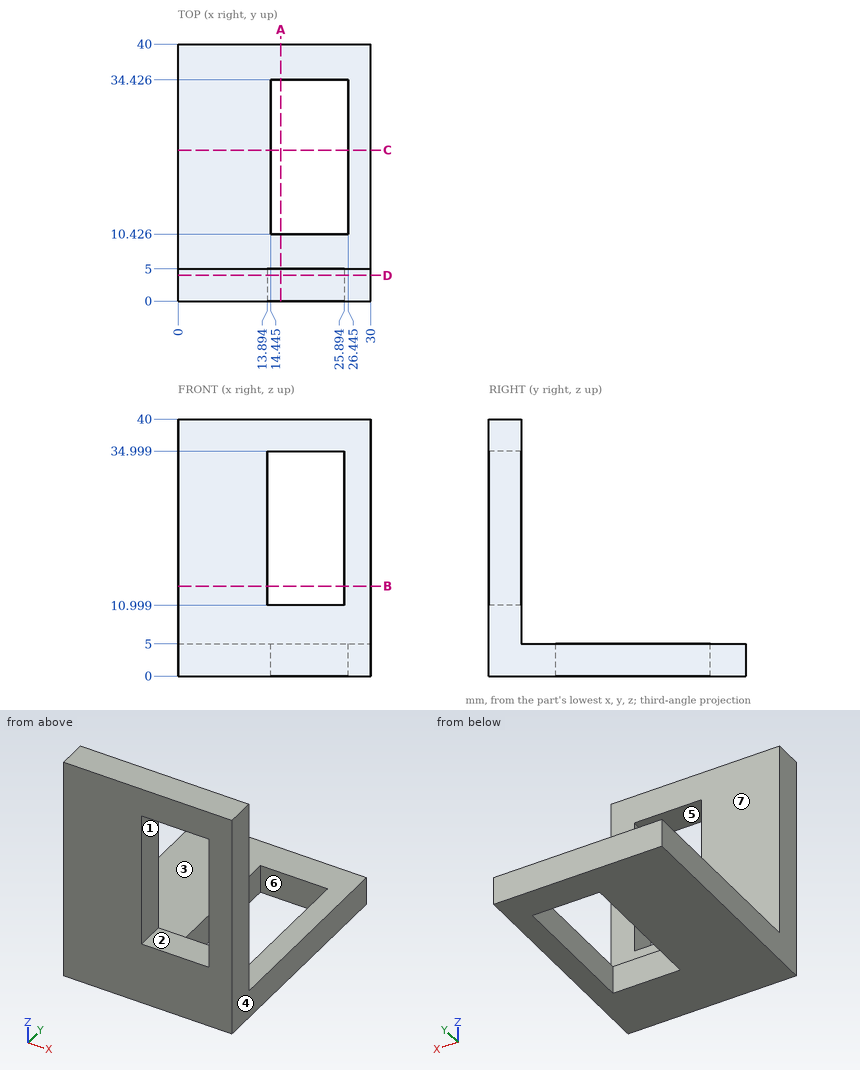
Geometry check sheet. Reference: drawing and pictorial views, mm from the part's lowest x, y, z. A direction names the side the tool comes from. Coordinates: 2 decimals unless noted, no trailing zeros. Loops run counter-clockwise (first coordinate to the right, second up) from the corner with the lowest first, then second, coordinate; pieces in that order, holes last. Notation, with made-up numbers: (-9, -13) -> (-1, -13) arc R27 cw to (-1, 22) -> close; hole circle Ø4 at (40, -2.75). An arc over 180 degrees is marked (long way). Put each result on its own line as item: value.
1) Cross-section at B-B on z = 14. Record the boundary of the cut face in (x, y).
Result set:
outline: (0, 0) -> (13.89, 0) -> (13.89, 5) -> (0, 5) -> close; (25.89, 0) -> (30, 0) -> (30, 5) -> (25.89, 5) -> close
2) Cross-section at C-C on y = 23.5. Record the boundary of the cut face in (x, z) (1 decimal).
Result set:
outline: (0, 0) -> (14.4, 0) -> (14.4, 5) -> (0, 5) -> close; (26.4, 0) -> (30, 0) -> (30, 5) -> (26.4, 5) -> close
3) Cross-section at D-D on y = 4. Record the boundary of the cut face in (x, z).
Result set:
outline: (0, 0) -> (30, 0) -> (30, 40) -> (0, 40) -> close; hole (13.89, 11) -> (25.89, 11) -> (25.89, 35) -> (13.89, 35) -> close
4) Thickness scan on line 1 (X direction, y = 3, z = 15.5); line 2 (Y direction, x = 11, z = 38); line 3 (X direction, y = 16.5, z = 2.5) (1 decimal). Record the ranges inside material, lowest first.
Result set:
line 1: x = 0 to 13.89, 25.89 to 30
line 2: y = 0 to 5
line 3: x = 0 to 14.4, 26.4 to 30
5) Cross-section at A-A on x = 16. Record the boundary of the cut face in (y, z), plus the area to 3 significant figures.
Result set:
outline: (0, 0) -> (10.43, 0) -> (10.43, 5) -> (5, 5) -> (5, 11) -> (0, 11) -> close; (0, 35) -> (5, 35) -> (5, 40) -> (0, 40) -> close; (34.43, 0) -> (40, 0) -> (40, 5) -> (34.43, 5) -> close
area: 135 mm^2
6) Tool access check on the marked faces 5, 6 and 7. Record the directions out of +Z, -Z, +X, -X, +Y, -Y that give a thin tool (end or side, any length) a straight path to the whole face; none if there is none.
Result set:
face 5: +Y, -Y
face 6: +Z, -Z
face 7: +Z, +X, -X, +Y
7) Gauge pin test, flat ends, axial feed: pin 1 Ø8 at (x, y) = (16, 32.5) entering from +Z; pin 2 Ø2 at (x, z) = (16.5, 13.5) entering from +Y. Record the tip position at first contact, or that the pin passes through.
Result set:
pin 1: stops at z = 5
pin 2: passes through
8) Release check for a two-part mould opening along Z. For the marked faces 1, 2, 3 and 4 record: released by +Z, released by -Z, zero draft, split by the parting line, or undercut.
Result set:
face 1: undercut
face 2: undercut
face 3: released by +Z
face 4: zero draft
